from build123d import *

# Parameters (mm, degrees)
F0_W     = 535
F0_H     = 800
F1_DEPTH = 14
F2_SIZE  = 13.99999


# Not quite as in the source:
# - a fillet or chamfer is up to 0.001 mm smaller than in the source, because OpenCascade refuses the exact size


with BuildPart() as f1:
    # F0 (on Right) → F1 (new body)
    with BuildSketch(Plane.YZ):
        Rectangle(F0_W, F0_H)
    extrude(amount=F1_DEPTH)

    # F2 (size 14 in the source; OpenCascade refuses exactly that, so slightly less here)
    f2_edges = [f1.edges().sort_by_distance(p)[0] for p in [
        (0, 0, 400),
        (0, 267.5, 0),
        (0, 0, -400),
    ]]
    chamfer(f2_edges, length=F2_SIZE)


solid = f1.part
Verification items for the finished model (mm, model axes). Coordinates: 2 decimals unless noted, no trailing zeros. Loops run counter-clockwise (first coordinate to the right, second up) from the corner with the lowest first, then second, coordinate; pieces in that order, holes last. Notation, with made-up numbers: (51, -39) -> (55, -39) arc R27 cw to (55, -12) -> close; hole circle Ø2 at (51, 30). An arc over 180 degrees is marked (long way). Answer as a JSON object with one key per item and string values. Group by question number.
Item 1: Depth check by flat-ended pin: pin 1 (5 mm diameter, centred on x = 6.5, y = 56.5, fed in from -Z); pin 2 (1 mm diameter, centred on x = 7.5, y = 45, fed in from -Z). Enter the tip coordinate at first touch or a pass-through.
Item 2: Sectioned sample at B-B on x = 5.75. Record the boundary of the cut face in (y, z).
Item 3: Scan lines: probe 1 along Y at (x, z) = (8.5, -33); probe 2 along Z at (x, y) = (13.5, -99); probe 3 along Y at (x, z) = (5.5, -188). Record each from-to range of solid material in increasing order.
Evaluation:
{
 "1": {"pin 1": "stops at z = -395", "pin 2": "stops at z = -394"},
 "2": {"outline": "(-267.5, -391.75) -> (259.25, -391.75) -> (259.25, 391.75) -> (-267.5, 391.75) -> close"},
 "3": {"probe 1": "y = -267.5 to 262", "probe 2": "z = -399.5 to 399.5", "probe 3": "y = -267.5 to 259"}
}
